Input: part model. Units: mm. Frame: model coordinates. A direction names the side the tool comes from. Coordinates: 2 decimals unless noted, no trailing zeros. Write each loop counter-clockwise with the first axis right and the second up, starting at its lowest first coordinate (ties: lowest second). Pieces come first, ordered by that corner, then holes.
1) Section query A-A (y = 59). Output: boundary loops of the cut face in (x, z), then the cut area to 3 significant figures.
2) Section query C-C (y = 41.5). Output: boundary loops of the cut face in (x, z), then the cut area to 3 significant figures.
3) Draft query along X for faces 1 (the flat face through (75, 15, 39)), 2 (the cylindrical face through (0.51, 79.998, 40.543)), 3 (the cylindrical face through (9.4, 57.8, 37.3)), 4 (the flat face through (-1, 31, 0)). Return one class per face: pulls with the +X half, pulls with the -X half, needs draft (parallel to the pull), parting line crosses it, or undercut.
4) Pin query (flat end, axial travel): pin 1 Ø23.5 at (x, z) = (58.5, 36) entering from +Y; pin 2 Ø1 at (y, z) = (53, 14) entering from -X; pin 3 Ø6 at (x, z) = (-13.5, 72) entering from +Y; pin 4 Ø6 at (x, y) = (59.5, 34) entering from -Z. Return the tip coordinate at first contact, or that it passes through.
5) Line query: L1, parallel to Y at x = 61, z = 64; L2, parallel to X at y = 55, z = 45.5; L3, parallel to X at y = 64, z = 25. Output: solid intervals per line, ascending.
6) Section query B-B (x = 65.5). Output: boundary loops of the cut face in (y, z).
7) Set-up query: faces 5 (the flat face through (57, 30, 31)), 6 (the flat face through (-1, 0, 39)), 7 (the flat face through (-57, 30, 48)). Return all of +Z, -Z, +X, -X, +Y, -Y with unobstructed straight access to the full face (end or side cutting, diameter ignored); none if empty.
from build123d import *

# Parameters (mm, degrees)
SKETCH1_W                       = 150
SKETCH1_H                       = 30
BOSS_EXTRUDE1_DEPTH             = 80
BOSS_EXTRUDE4_REACH             = 65.239
SKETCH3_R                       = 10
BOSS_EXTRUDE4_DIRECTION_2_REACH = 65.239


with BuildPart() as part:
    # Sketch1 → Boss-Extrude1 (new body)
    with BuildSketch(Plane.XY):
        with Locations((0, 15)):
            Rectangle(SKETCH1_W, SKETCH1_H)
    extrude(amount=BOSS_EXTRUDE1_DEPTH)

    # Boss-Extrude4: up to this face of the body (flat: up to its plane)
    boss_extrude4_end = Plane(part.part.faces().sort_by_distance((0, 15, 80))[0])
    # Sketch3 → Boss-Extrude4 (add, up to the picked face)
    with BuildSketch(Plane(origin=(12.855752194, 0, 35.320888862), x_dir=(0, 1, 0), z_dir=(0.342020143, 0, 0.939692621)), mode=Mode.PRIVATE) as boss_extrude4_sk1:
        with BuildLine():
            Line((30, -26.73371311), (70, -3.639702343))
            ThreePointArc((70, -3.639702343), (80, 13.680805733), (70, 31.001313809))
            Line((70, 31.001313809), (30, 54.095324576))
            Line((30, 54.095324576), (30, -26.73371311))
        make_face()
        with Locations((60, 13.680805733)):
            Circle(SKETCH3_R, mode=Mode.SUBTRACT)
    boss_extrude4_tool1 = split(extrude(boss_extrude4_sk1.sketch, amount=BOSS_EXTRUDE4_REACH, mode=Mode.PRIVATE), bisect_by=boss_extrude4_end, keep=Keep.BOTH, mode=Mode.PRIVATE)
    add(boss_extrude4_tool1.solids().sort_by_distance((0, 48.492065, 40))[0])

    # Boss-Extrude4 direction 2: up to this face of the body (flat: up to its plane)
    boss_extrude4_direction_2_end = Plane(part.part.faces().sort_by_distance((0, 15, 0))[0])
    # Sketch3 → Boss-Extrude4 direction 2 (add, up to the picked face)
    with BuildSketch(Plane(origin=(12.855752194, 0, 35.320888862), x_dir=(0, 1, 0), z_dir=(0.342020143, 0, 0.939692621)), mode=Mode.PRIVATE) as boss_extrude4_direction_2_sk1:
        with BuildLine():
            Line((30, -26.73371311), (70, -3.639702343))
            ThreePointArc((70, -3.639702343), (80, 13.680805733), (70, 31.001313809))
            Line((70, 31.001313809), (30, 54.095324576))
            Line((30, 54.095324576), (30, -26.73371311))
        make_face()
        with Locations((60, 13.680805733)):
            Circle(SKETCH3_R, mode=Mode.SUBTRACT)
    boss_extrude4_direction_2_tool1 = split(extrude(boss_extrude4_direction_2_sk1.sketch, amount=-BOSS_EXTRUDE4_DIRECTION_2_REACH, mode=Mode.PRIVATE), bisect_by=boss_extrude4_direction_2_end, keep=Keep.BOTH, mode=Mode.PRIVATE)
    add(boss_extrude4_direction_2_tool1.solids().sort_by_distance((0, 48.492065, 40))[0])


solid = part.part
Answer:
1. outline: (-39.75, 0) - (-25.15, 0) - (3.97, 80) - (-10.63, 80) - close; (-3.97, 0) - (10.63, 0) - (39.75, 80) - (25.15, 80) - close
1. area: 2,340 mm2
2. outline: (-50.5, 0) - (21.38, 0) - (50.5, 80) - (-21.38, 80) - close
2. area: 5,750 mm2
3. face 1: pulls with the +X half
3. face 2: parting line crosses it
3. face 3: undercut
3. face 4: needs draft
4. pin 1: stops at y = 30
4. pin 2: stops at x = -38.7
4. pin 3: stops at y = 64.27
4. pin 4: passes through
5. L1: y = 0 to 30
5. L2: x = -25.65 to -7.21, 11.22 to 29.65
5. L3: x = -27.58 to -15.21, 4.29 to 16.66
6. outline: (0, 0) - (30, 0) - (30, 80) - (0, 80) - close
7. face 5: -Z, +X, +Y
7. face 6: +Z, -Z, +X, -X, -Y
7. face 7: +Z, -X, +Y
